Autodesk Inventor part; units mm, degrees
ref_plane "Work Plane1" through (0, 2, 4) normal (1, 0, 0) x (0, 0, -1)
ref_plane "YZ Plane" through (0, 0, 0) normal (1, 0, 0) x (0, 1, 0)
ref_plane "XZ Plane" through (0, 0, 0) normal (0, 1, 0) x (-1, 0, 0)
sketch "Sketch1" plane through (0, 0, 0) normal (0, 1, 0) x (-1, 0, 0)
  line L0 (24.5, 6) -> (0, 6)
  line L1 (0, 6) -> (0, 0)
  line L2 (0, 0) -> (24.5, 0)
  line L3 (24.5, 0) -> (24.5, 6)
  circle A0 centre (24.5, 3) radius 3
  circle A1 centre (24.5, 3) radius 1
  line L4 (22.2639, 1) -> (0, 1)
  line L5 (0, 1) -> (0, 0)
  line L6 (0, 0) -> (22.2639, 0)
  line L7 (22.2639, 0) -> (22.2639, 1)
  line L8 (0, 4) -> (15.5, 4)
  line L9 (15.5, 4) -> (15.5, 1)
  line L10 (15.5, 1) -> (0, 1)
  line L11 (0, 1) -> (0, 4)
  line L12 (24.5, 3) -> (0, 3)
  line L13 (0, 3) -> (0, 7)
  line L14 (0, 7) -> (24.5, 7)
  line L15 (24.5, 7) -> (24.5, 3)
  line L16 (24.5, 7) -> (20.5, 7)
  line L17 (20.5, 7) -> (20.5, 6)
  line L18 (20.5, 6) -> (24.5, 6)
  line L19 (24.5, 6) -> (24.5, 7)
  circle A2 centre (22.5, 8) radius 2
  line L20 (15.5, 4) -> (15.5, 7)
  point P0 (22.5, 6)
  point P1 (20.7679, 7)
  point P2 (0, 6)
  point P3 (15.5, 3)
  point P4 (0, 3)
  point P5 (15.5, 6)
  point P6 (0, 6)
  dimension "d0" = 24.5
  dimension "d1" = 6
  dimension "d2" = 2
  dimension "d3" = 0
  dimension "d4" = 0
  dimension "d6" = 3
  dimension "d7" = 4
  dimension "d8" = 4
  dimension "d9" = 4
  dimension "d10" = 2
  dimension "d13" = 2
  dimension "d14" = 9
extrude "Extrusion1" add sketch "Sketch1" along normal blind 2 contours A0 L12 L9 L20 L0 | A0 L3 A1 | L3 A1 L12 A0 | L0 L17 L14 A2 | L12 A1 L3 A0 | A0 L4 L9 L12 | L0 L20 L14 L17 | L20 L8 L1 L0 | L0 L13 L14 L20
sketch "Sketch2" plane through (0, 0, 7) normal (1, 0, 0) x (0, 0, -1)
  line L0 (0, 2) -> (3, 2)
  line L1 (3, 2) -> (0, 2)
  line L2 (0, 2) -> (0, 12)
  line L3 (0, 12) -> (3, 12)
  line L4 (3, 12) -> (3, 2)
  line L5 (0, 12) -> (12, 12)
  line L6 (12, 12) -> (12, 9)
  line L7 (12, 9) -> (0, 9)
  line L8 (0, 9) -> (0, 12)
  line L9 (0, 0) -> (3, 0)
  circle A0 centre (10.5, 4.5) radius 7.5
  line L10 (3, 2) -> (6, 2)
  line L11 (0, 12) -> (12, 12)
  line L12 (12, 12) -> (12, 14)
  line L13 (12, 14) -> (0, 14)
  line L14 (0, 14) -> (0, 12)
  circle A1 centre (10.5, 4.5) radius 9.5
  line L15 (0, 2) -> (1.3214, 6.9501)
  point P0 (7, 0)
  point P1 (10.5, 14)
  point P2 (3, 4.5)
  point P3 (10.5, 12)
  dimension "d15" = 10
  dimension "d16" = 12
  dimension "d17" = 3
  dimension "d20" = 15
  dimension "d21" = 2.5
  dimension "d22" = 7.5
  dimension "d23" = 12
  dimension "d24" = 2
extrude "Extrusion2" add sketch "Sketch2" against normal blind 15 contours L15 A1 L0 | A1 L7 L4 L0 | A1 L4 L7 | L4 L7 A0 | L4 A1 L5 A0 L7 | A1 L13 L12 | L12 L5 A1
mirror "Mirror1" about plane through (0, 0, 7) normal (1, 0, 0) of "Extrusion1", "Extrusion2"
ref_plane "Work Plane1" through (0, 2, 4) normal (1, 0, 0) x (0, 0, -1)
sketch "Sketch4" plane through (0, 2, 4) normal (1, 0, 0) x (0, 0, -1)
  line L0 (-3, 0) -> (-1.6786, 4.9501)
  line L1 (-3, 0) -> (-3, 4.9501)
  line L2 (-3, 4.9501) -> (-1.6786, 4.9501)
  arc A0 (7.5, 12) -> (-1.6786, 4.9501) centre (7.5, 2.5) ccw
  arc A1 (7.5, 12) -> (-3, 4.9501) centre (7.0292, 1.357) ccw
  circle A2 centre (7.5, 2.5) radius 9.5
  point P0 (4, -2)
extrude "Extrusion3" add sketch "Sketch4" along normal mid plane 2 contours L1 L2 L0 | L2 A1 A0
pattern_linear "Rectangular Pattern1" count 2 spacing 14 along (-1, 0, 0) count 2 spacing 14 along (1, 0, 0) of "Extrusion3"
sketch "Sketch5" plane through (-15, 0, 7) normal (-1, 0, 0) x (0, 0, 1)
  point P0 (-7, 0)
equation "\"d11\" = d2"
properties part number "Battery mount front"
Verification items for the finished model (mm, model axes). A direction names the side the tool comes from. Coordinates: 2 decimals unless noted, no trailing zeros. Order: outer loops, then holes, each group sorted by start corner. A loop starts at its lowest first (then second) coordinate and runs counter-clockwise, first axis right, second up.
1. Sectioned sample at A-A, the plane z = 2.5. Record the cut outline in (x, y).
Results found:
outline: (-27.46, 0) - (-25.37, 0) - (-25.37, 2) - (-27.46, 2) - close; (-23.63, 0) - (-15.5, 0) - (-15.5, 2) - (-23.63, 2) - close; (-15, 9) - (15, 9) - (15, 12.46) - (13, 12.46) - (13, 11.87) - (1, 11.87) - (1, 12.46) - (-1, 12.46) - (-1, 11.87) - (-13, 11.87) - (-13, 12.46) - (-15, 12.46) - close; (15.5, 0) - (23.63, 0) - (23.63, 2) - (15.5, 2) - close; (25.37, 0) - (27.46, 0) - (27.46, 2) - (25.37, 2) - close
2. Sectioned sample at C-C, the plane x = -24. Record the cut outline in (y, z), and give its area (3 significant figures).
Results found:
outline: (0, 0.04) - (2, 0.04) - (2, 2.13) - (0, 2.13) - close; (0, 3.87) - (2, 3.87) - (2, 6) - (0, 6) - close
area: 8.45 mm2
3. Release check for a two-part mould opening along X. For faces 1 (the face through (-21.51, 0.99, 6.26)), 2 (the face through (-15.5, 1, 3)), 3 (the face through (15, 9, 3)), 4 (the face through (0, 12, -4)) record: +X half, -X half, draft (parallel to the pull), parting line (faces both ways), or undercut.
Results found:
face 1: -X half
face 2: undercut
face 3: +X half
face 4: draft
4. Set-up check for faces 5 (the face through (-24, 1, 6)), 6 (the face through (19, 1, 1)), 7 (the face through (13, 8.5, 5.3)): record each of +Z, -Z, +X, -X, +Y, -Y from which the full face is reachable in a straight line by a thin tool's end or side.
Results found:
face 5: +Z, -X, +Y, -Y
face 6: -Z, +Y, -Y
face 7: +Z, +Y
5. Go/stop test with flat-tipped pins: pin 1 Ø0.6 at (x, y) = (20.5, 1) entering from -Z; pin 2 Ø1 at (y, z) = (12, 0) entering from +X; pin 3 Ø5.5 at (x, z) = (-23.5, 4.5) entering from +Y; pin 4 Ø1.2 at (x, z) = (-24.5, 3) entering from -Y. Record where each tip stops, or that it passes through.
Results found:
pin 1: stops at z = 1
pin 2: stops at x = 15
pin 3: stops at y = 2
pin 4: passes through
6. Scan lines: line 1 (X direction, y = 1.6, z = 3); line 2 (Z direction, x = -24.5, y = 1.6); line 3 (Z direction, x = 0.5, y = 2.25). Record each from-to range of solid material in increasing order.
Results found:
line 1: x = -27.5 to -25.5, -23.5 to -15.5, 15.5 to 23.5, 25.5 to 27.5
line 2: z = 0 to 2, 4 to 6
line 3: z = 4 to 7
7. Sectioned sample at B-B, the plane x = -6. Record the cut outline in (y, z).
Results found:
outline: (0, 4) - (4.5, 4) arc R7.5 cw to (12, -3.5) - (12, -5) - (14, -5) - (14, -3.5) arc R9.5 ccw to (6.95, 5.68) - (2, 7) - (0, 7) - close
8. Sectioned sample at D-D, the plane y = 11.5. Record the cut outline in (x, z), and give its area (3 significant figures).
Results found:
outline: (-15, -0.81) - (15, -0.81) - (15, 3.84) - (13, 3.84) - (13, 2.92) - (1, 2.92) - (1, 3.84) - (-1, 3.84) - (-1, 2.92) - (-13, 2.92) - (-13, 3.84) - (-15, 3.84) - close
area: 117 mm2
